from build123d import *

# Parameters (mm, degrees)
SKETCH2_R           = 2.5
BOSS_EXTRUDE1_DEPTH = 34
SKETCH3_R           = 2.5
BOSS_EXTRUDE2_DEPTH = 17


with BuildPart() as part:
    # Sketch2 → Boss-Extrude1 (new body)
    with BuildSketch(Plane(origin=(0, 0, 0), x_dir=(1, 0, 0), z_dir=(0, 1, 0))):
        Circle(SKETCH2_R)
    extrude(amount=BOSS_EXTRUDE1_DEPTH)

    # Sketch3 → Boss-Extrude2 (add, symmetric)
    with BuildSketch(Plane(origin=(0, 0, 0), x_dir=(0, 0, -1), z_dir=(1, 0, 0))):
        with Locations((0, 17)):
            Circle(SKETCH3_R)
    extrude(amount=BOSS_EXTRUDE2_DEPTH, both=True)


solid = part.part
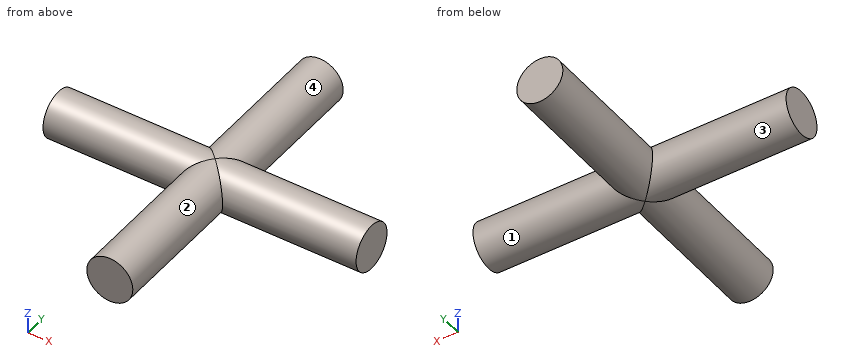
Here's how the part is built. I have some questions about the finished solid (model axes, mm). Face numbers are marked on the shaded views. A direction names the side the tool comes from. Round coordinates to 2 decimals unless told otherwise and drop trailing zeros. Write each loop counter-clockwise with the first axis right and the second up, starting at its lowest first coordinate (ties: lowest second). Pieces come first, ordered by that corner, then holes.
1. Suppose I cut it at A-A (z = -1.15). List the corners of the cut face in (x, y) for me, and give its area (3 significant figures).
2. Suppose I cut it at B-B (y = 31). List the corners of the cut face in (x, z) for me, and give its area (3 significant figures).
3. For the marked faces 1, 2, 3 and 4, which set-ups out of +Z, -Z, +X, -X, +Y, -Y let a thin tool reach every point of the face, with its end or its side?
4. Will these pins go through, and if not, where does the flat tip stop? pin 1 Ø5 at (x, y) = (4.5, 10) entering from -Z; pin 2 Ø1.5 at (x, z) = (-6, -1.5) entering from +Y.
5. Suppose I cut it at D-D (y = 16.5). List the corners of the cut face in (x, z) for me.
6. I need wall thicknesses on L1, parallel to Z at x = -15, y = 16.5; L2, parallel to Y at x = 13, z = 2.25; L3, parallel to X at y = 21.5, z = -1.65. Which ranges of each line are inside material? Lowest first, please.
7. Suppose I cut it at C-C (x = -1). List the corners of the cut face in (y, z) for me, and give its area (3 significant figures).
Answer sheet:
1. outline: (-17, 14.78) - (-2.22, 14.78) - (-2.22, 0) - (2.22, 0) - (2.22, 14.78) - (17, 14.78) - (17, 19.22) - (2.22, 19.22) - (2.22, 34) - (-2.22, 34) - (-2.22, 19.22) - (-17, 19.22) - close
1. area: 282 mm2
2. outline: circle Ø5 at (0, 0)
2. area: 19.6 mm2
3. face 1: +X
3. face 2: -Y
3. face 3: -X
3. face 4: +Y
4. pin 1: stops at z = -1.5
4. pin 2: stops at y = 19.38
5. outline: (-17, -2.45) - (-0.5, -2.45) arc R2.5 ccw to (0.5, -2.45) - (17, -2.45) - (17, 2.45) - (0.5, 2.45) arc R2.5 ccw to (-0.5, 2.45) - (-17, 2.45) - close
6. L1: z = -2.45 to 2.45
6. L2: y = 15.91 to 18.09
6. L3: x = -1.88 to 1.88
7. outline: (0, -2.29) - (16, -2.29) arc R2.5 ccw to (18, -2.29) - (34, -2.29) - (34, 2.29) - (18, 2.29) arc R2.5 ccw to (16, 2.29) - (0, 2.29) - close
7. area: 156 mm2
